Model file for the job. Use its own axes, mm. Face numbers are marked on the shaded views. A direction names the side the tool comes from. Give positions to 0.01 mm unless a question says otherwise; leave off trailing zeros. Loops run counter-clockwise (first coordinate to the right, second up) from the corner with the lowest first, then second, coordinate; pieces in that order, holes last. Notation, with made-up numbers: M -37,23.5 L -21,23.5 A17 cw -21,51.5 Z; hole C 78,0.5 d4. An arc over 180 degrees is marked long. Use CSV: the item, a comma, the result in double quotes. Start each with the question number.
(1) Slice it at B-B on y = 7.5. List the corners of the cut face in (x, z), and give its area (3 significant figures).
(2) Two-plate mould, pull along Z, no slides. Class the marked faces 3, 4 and 5: pulls with the +Z half, pulls with the -Z half, needs draft (parallel to the pull), parting line crosses it, or undercut.
(3) Slice it at D-D on x = -19.5. List the corners of the cut face in (y, z).
(4) Wall check: line 1 along X through (y, z) = (7.5, 39); line 2 along Z through (x, y) = (18.5, 22.5); line 3 along X through (y, z) = (28.5, 51). Give the ranges that are in metal, low to high. Write a range as from..to.
(5) Slice it at C-C on x = -0.5. List the corners of the cut face in (y, z), and give its area (3 significant figures).
(6) Tool access for the marked faces 1 and 2: list every direction of +Z, -Z, +X, -X, +Y, -Y with a clear straight run to the whole face (end or side of a thin tool).
(7) Flat gauge pins, fed straight in: P1, Ø1, axis at x = 25.5, y = 29, coming from the +Z side; P2, Ø4, axis at x = 0, z = 21, coming from the +Y side; P3, Ø1.6, axis at y = 15.5, z = -54.5, coming from the +X side. Where does each tip first touch, or does it go through?
(8) Slice it at A-A on z = 45. List the corners of the cut face in (x, y), and give its area (3 significant figures).
Autodesk Inventor part; units mm, degrees
ref_plane "YZ Plane" through (0, 0, 0) normal (1, 0, 0) x (0, 1, 0)
ref_plane "XZ Plane" through (0, 0, 0) normal (0, 1, 0) x (-1, 0, 0)
ref_plane "XY Plane" through (0, 0, 0) normal (0, 0, 1) x (1, 0, 0)
sketch "Sketch1" plane through (0, 0, 0) normal (0, 1, 0) x (-1, 0, 0)
  line L0 (-19.5, -45) -> (19.5, -45) construction
  line L1 (19.5, -45) -> (19.5, 45) construction
  line L2 (19.5, 45) -> (-19.5, 45) construction
  line L3 (-19.5, 45) -> (-19.5, -45) construction
  line L4 (-19.5, -45) -> (19.5, 45) construction
  line L5 (19.5, -45) -> (-19.5, 45) construction
  line L6 (-27, -55) -> (27, -55)
  line L7 (27, -55) -> (27, 55)
  line L8 (27, 55) -> (-27, 55)
  line L9 (-27, 55) -> (-27, -55)
  line L10 (-27, -55) -> (27, 55) construction
  line L11 (27, -55) -> (-27, 55) construction
  circle A0 centre (19.5, 45) radius 1.45
  circle A1 centre (-19.5, 45) radius 1.45
  circle A2 centre (19.3553, -44.6662) radius 1.45
  circle A3 centre (-19.5, -45) radius 1.45
  point P0 (0, 0)
  dimension "d0" = 39
  dimension "d1" = 90
  dimension "d2" = 54
  dimension "d3" = 110
  dimension "d4" = 2.9
  dimension "d5" = 2.9
  dimension "d6" = 2.9
  dimension "d7" = 2.9
extrude "Extrusion1" add sketch "Sketch1" along normal blind 3
fillet "Fillet1" radius 5 4 edges at (27, 1.5, 55) (-27, 1.5, 55) (-27, 1.5, -55) (27, 1.5, -55)
sketch "Sketch2" plane through (0, 3, 0) normal (0, 1, 0) x (1, 0, 0)
  arc A0 (27, 50) -> (22, 55) centre (22, 50) ccw
  line L0 (22, 55) -> (-22, 55)
  arc A1 (-22, 55) -> (-27, 50) centre (-22, 50) ccw
  line L1 (-27, 50) -> (-27, -50)
  arc A2 (-27, -50) -> (-22, -55) centre (-22, -50) ccw
  line L2 (-22, -55) -> (22, -55)
  arc A3 (22, -55) -> (27, -50) centre (22, -50) ccw
  line L3 (27, -50) -> (27, 50)
  circle A4 centre (19.5, 45) radius 1.45
  circle A5 centre (-19.3553, 44.6662) radius 1.45
  circle A6 centre (19.5, -45) radius 1.45
  circle A7 centre (-19.5, -45) radius 1.45
  line L4 (-25, -50) -> (-25, 50)
  arc A8 (-22, 53) -> (-25, 50) centre (-22, 50) ccw
  line L5 (-22, 53) -> (22, 53)
  arc A9 (25, 50) -> (22, 53) centre (22, 50) ccw
  line L6 (25, 50) -> (25, -50)
  arc A10 (22, -53) -> (25, -50) centre (22, -50) ccw
  line L7 (22, -53) -> (-22, -53)
  arc A11 (-25, -50) -> (-22, -53) centre (-22, -50) ccw
  point P0 (0, 0)
  dimension "d11" = 2
extrude "Extrusion2" add sketch "Sketch2" along normal blind 30 contours L3 A3 L2 A2 L1 A1 L0 A0
sketch "Sketch3" plane through (-22, 0, 55) normal (0, 0, 1) x (1, 0, 0)
  line L0 (41, 18) -> (26, 18)
  line L1 (26, 18) -> (26, 10)
  line L2 (26, 10) -> (41, 10)
  line L3 (41, 10) -> (41, 18)
  line L4 (41, 18) -> (26, 10) construction
  line L5 (26, 18) -> (41, 10) construction
  line L6 (49, 0) -> (49, 33)
  line L7 (0, 0) -> (44, 0)
  point P0 (22, 0)
  point P1 (33.5, 14)
  dimension "d14" = 8
  dimension "d15" = 10
  dimension "d16" = 15
  dimension "d17" = 8
extrude "Extrusion3" cut sketch "Sketch3" against normal blind 30
sketch "Sketch4" plane through (22, 0, -55) normal (0, 0, -1) x (-1, 0, 0)
  line L0 (0, 0) -> (0, 33)
  line L1 (0, 0) -> (44, 0)
  line L2 (44, 33) -> (44, 0)
  line L3 (0, 33) -> (44, 33)
  line L4 (18, 10) -> (18, 18) construction
  line L5 (18, 18) -> (3, 18) construction
  line L6 (3, 18) -> (3, 10) construction
  line L7 (3, 10) -> (18, 10) construction
  line L8 (44, 0) -> (44, 33) construction
  line L9 (44, 0) -> (0, 0) construction
  line L10 (0, 33) -> (0, 0) construction
  line L11 (44, 33) -> (0, 33) construction
  line L12 (3, 10) -> (38, 10)
  line L13 (38, 10) -> (38, 18)
  line L14 (38, 18) -> (3, 18)
  line L15 (3, 18) -> (3, 10)
  point P0 (22, 0)
  dimension "d20" = 35
extrude "Extrusion4" cut sketch "Sketch4" against normal blind 30 contours L15 L14 L13 L12
sketch "Sketch5" plane through (0, 33, 0) normal (0, 1, 0) x (1, 0, 0)
  arc A0 (-25, -50) -> (-22, -53) centre (-22, -50) ccw
  arc A1 (22, -53) -> (25, -50) centre (22, -50) ccw
  arc A2 (25, 50) -> (22, 53) centre (22, 50) ccw
  arc A3 (-22, 53) -> (-25, 50) centre (-22, 50) ccw
  circle A4 centre (-23, -51) radius 1.45
  circle A5 centre (23, -51) radius 1.45
  circle A6 centre (-23, 51) radius 1.45
  arc A7 (-22, 53) -> (-25, 50) centre (-22, 50) ccw
  line L0 (-22, 53) -> (22, 53)
  arc A8 (25, 50) -> (22, 53) centre (22, 50) ccw
  line L1 (25, 50) -> (25, -50)
  arc A9 (22, -53) -> (25, -50) centre (22, -50) ccw
  line L2 (22, -53) -> (-22, -53)
  arc A10 (-25, -50) -> (-22, -53) centre (-22, -50) ccw
  line L3 (-25, -50) -> (-25, 50)
  arc A11 (27, 50) -> (22, 55) centre (22, 50) ccw
  line L4 (22, 55) -> (-22, 55)
  arc A12 (-22, 55) -> (-27, 50) centre (-22, 50) ccw
  line L5 (-27, 50) -> (-27, -50)
  arc A13 (-27, -50) -> (-22, -55) centre (-22, -50) ccw
  line L6 (-22, -55) -> (22, -55)
  arc A14 (22, -55) -> (27, -50) centre (22, -50) ccw
  line L7 (27, -50) -> (27, 50)
  arc A15 (-22, 51) -> (-23, 50) centre (-22, 50) ccw construction
  line L8 (-22, 51) -> (22, 51) construction
  arc A16 (23, 50) -> (22, 51) centre (22, 50) ccw construction
  line L9 (23, 50) -> (23, -50) construction
  arc A17 (22, -51) -> (23, -50) centre (22, -50) ccw construction
  line L10 (22, -51) -> (-22, -51) construction
  arc A18 (-23, -50) -> (-22, -51) centre (-22, -50) ccw construction
  line L11 (-23, -50) -> (-23, 50) construction
  line L12 (23, 51) -> (-23, 51) construction
  line L13 (-23, 51) -> (-23, -51) construction
  line L14 (-23, -51) -> (23, -51) construction
  line L15 (23, -51) -> (23, 51) construction
  line L16 (23, 51) -> (-23, -51) construction
  line L17 (-23, 51) -> (23, -51) construction
  line L18 (-25, 50) -> (-25, -50)
  arc A19 (-22, -53) -> (-25, -50) centre (-22.8913, -50.8913) ccw
  line L19 (-22, -53) -> (22, -53)
  arc A20 (25, -50) -> (22, -53) centre (22.921, -50.921) ccw
  arc A21 (-25, 50) -> (-22, 53) centre (-22.9063, 50.9063) ccw
  arc A22 (25, 50) -> (22, 53) centre (22, 50) ccw
  arc A23 (22, 53) -> (25, 50) centre (22.4561, 50.4561) ccw
  circle A24 centre (22.4561, 50.4561) radius 1.45
  circle A25 centre (-23, -51) radius 2.2361
  circle A26 centre (23, -51) radius 2.2361
  point P0 (0, 0)
  point P1 (24.1213, 52.1213)
  dimension "d23" = 2.9
  dimension "d24" = 2.9
  dimension "d25" = 2.9
  dimension "d27" = 2
  dimension "d28" = 2.9
extrude "Extrusion5" add sketch "Sketch5" against normal blind 10 contours A26 A1 | A1 A26 | A2 A23
ref_plane "Work Plane1" through (22, 3, 50) normal (0, 0, -1) x (-1, 0, 0)
sketch "Sketch6" plane through (22, 3, 50) normal (0, 0, -1) x (-1, 0, 0)
  line L0 (46.829, 28.3524) -> (47.7477, 28.3524)
  line L1 (47.7477, 28.3524) -> (46.829, 24.7431)
  line L2 (46.829, 24.7431) -> (46.829, 28.3524)
  line L3 (22, 24.0878) -> (22, -17.3662)
  line L4 (-2.829, 28.3524) -> (-3.7477, 28.3524)
  line L5 (-3.7477, 28.3524) -> (-2.829, 24.7431)
  line L6 (-2.829, 24.7431) -> (-2.829, 28.3524)
  point P0 (22, -3)
extrude "Extrusion6" cut sketch "Sketch6" along normal blind 100
properties part number "00_Case_Powersupply_Galvo"
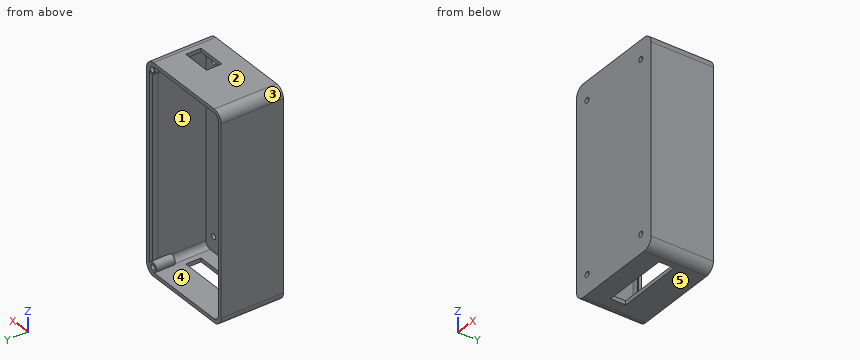
Reply:
1,outline,"M -27,-50 A5 ccw -22,-55 L 22,-55 A5 ccw 27,-50 L 27,50 A5 ccw 22,55 L -22,55 A5 ccw -27,50 Z; hole M -25,-50 A3 ccw -22,-53 L 22,-53 A3 ccw 25,-50 L 25,50 A3 ccw 22,53 L -22,53 A3 ccw -25,50 Z"
1,area,"626 mm^2"
2,face 3,"pulls with the +Z half"
2,face 4,"undercut"
2,face 5,"pulls with the -Z half"
3,outline,"M 0,-55 L 33,-55 L 33,-53 L 3,-53 L 3,-46.11 L 0,-46.11 Z; M 0,-43.22 L 3,-43.22 L 3,43.55 L 0,43.55 Z; M 0,46.45 L 3,46.45 L 3,53 L 33,53 L 33,55 L 0,55 Z"
4,line 1,"x = -27..-25, 25..27"
4,line 2,"z = -55..-53, 53..55"
4,line 3,"x = -26.9..-24.83, 20.76..21.55, 24.45..26.9"
5,outline,"M 0,-55 L 10,-55 L 10,-53 L 3,-53 L 3,53 L 33,53 L 33,55 L 0,55 Z; M 18,-55 L 33,-55 L 33,-53 L 18,-53 Z"
5,area,"434 mm^2"
6,face 1,"+Y"
6,face 2,"+Z, +X, -X, +Y, -Y"
7,P1,"stops at z = 54"
7,P2,"stops at y = 3"
7,P3,"stops at x = 25.36"
8,outline,"M -27,0 L -20.95,0 L -20.95,3 L -25,3 L -25,28.41 L -25.75,31.35 L -25,31.35 L -25,33 L -27,33 Z; M -18.05,0 L 18.05,0 L 18.05,3 L -18.05,3 Z; M 20.95,0 L 27,0 L 27,33 L 25,33 L 25,31.35 L 25.75,31.35 L 25,28.41 L 25,3 L 20.95,3 Z"
8,area,"262 mm^2"
